Design review of the part built by this model. Coordinates are the model's own, in mm. A direction names the side the tool comes from. Coordinates: 2 decimals unless noted, no trailing zeros. Write each loop counter-clockwise with the first axis right and the second up, starting at its lowest first coordinate (ties: lowest second). Pieces come first, ordered by that corner, then holes.
Q1. Insertion check: pin 1 (2.5 mm diameter, centred on y = 2.5, z = 33.5, fed in from +X); pin 2 (2.5 mm diameter, centred on y = 3, z = -30.5, fed in from +X); pin 3 (0.9 mm diameter, centred on x = -44, z = 25.5, fed in from -Y). Each pin has a flat end and moves straight along its axis. Give the tip position at first contact, or say it passes through.
Q2. Take a section at D-D (y = 1.5). State how many separate pieces and enclosed holes the cut face has, and give its area (3 significant figures).
Q3. Machinability: for faces 1 (the cylindrical face through (-0.325, 1.232, 52.464)), 2 (the cylindrical face through (5.94, 2.46, 42.93)), which of the approach directions +Z, -Z, +X, -X, +Y, -Y give a long, thin tool a straight path to every point of the face, cutting with its end or side? Answer none if there is none.
Q4. Take a section at C-C (z = 19). Give the boundary of the cut face in (x, y).
Q5. Take a section at B-B (x = -30). Give the boundary of the cut face in (y, z).
Q6. For probe 1 along Z at (x, y) = (0, 1.2); probe 2 along X at (y, z) = (4.75, -24); probe 3 along Z at (x, y) = (20, 4.75), list the stretches that pass through material, from the lowest coordinate up.
Q7. Take a section at A-A (x = 0). Give the boundary of the cut face in (y, z), and give its area (3 significant figures).
Q8. Mouldability with a two-part tool opening along X and no side actions: class faces 3 (the cylindrical face through (4.956, 2.465, 23.257)), 4 (the flat face through (-1, 0, -13)) as pulls with the +X half, pulls with the -X half, needs draft (parallel to the pull), parting line crosses it, or undercut.
```python
from build123d import *

# Parameters (mm, degrees)
SKETCH1_R           = 55
BOSS_EXTRUDE1_DEPTH = 5
SKETCH2_R           = 1.5
CUT_EXTRUDE1_DEPTH  = 2.5
SKETCH5_R           = 12.7
CUT_EXTRUDE4_DEPTH  = 6
CUT_EXTRUDE5_DEPTH  = 6
FILLET1_R           = 5
FILLET2_R           = 5


with BuildPart() as part:
    # Sketch1 → Boss-Extrude1 (new body)
    with BuildSketch(Plane(origin=(0, 0, 0), x_dir=(1, 0, 0), z_dir=(0, 1, 0))):
        Circle(SKETCH1_R)
    extrude(amount=BOSS_EXTRUDE1_DEPTH)

    # Sketch2 → Cut-Extrude1 (cut)
    with BuildSketch(Plane(origin=(0, 0, 0), x_dir=(1, 0, 0), z_dir=(0, 1, 0))):
        with Locations((0, 51)):
            Circle(SKETCH2_R)
        with Locations((44.167295593, 25.5)):
            Circle(SKETCH2_R)
        with Locations((44.167295593, -25.5)):
            Circle(SKETCH2_R)
        with Locations((0, -51)):
            Circle(SKETCH2_R)
        with Locations((-44.167295593, -25.5)):
            Circle(SKETCH2_R)
        with Locations((-44.167295593, 25.5)):
            Circle(SKETCH2_R)
    extrude(amount=CUT_EXTRUDE1_DEPTH, mode=Mode.SUBTRACT)

    # Sketch5 → Cut-Extrude4 (cut, through all)
    with BuildSketch(Plane(origin=(0, 5, 0), x_dir=(1, 0, 0), z_dir=(0, 1, 0))):
        Circle(SKETCH5_R)
    extrude(amount=-CUT_EXTRUDE4_DEPTH, mode=Mode.SUBTRACT)

    # Sketch7 → Cut-Extrude5 (cut, through all)
    with BuildSketch(Plane(origin=(0, 5, 0), x_dir=(1, 0, 0), z_dir=(0, 1, 0))):
        with BuildLine():
            Line((-21.351162756, 7.708297411), (-40.816877772, 18.946833216))
            ThreePointArc((-40.816877772, 18.946833216), (-45, 0), (-40.816877772, -18.946833216))
            Line((-40.816877772, -18.946833216), (-21.351162756, -7.708297411))
            ThreePointArc((-21.351162756, -7.708297411), (-22.7, 0), (-21.351162756, 7.708297411))
        make_face()
        with BuildLine():
            Line((-17.351162756, -14.636500641), (-36.816877772, -25.875036446))
            ThreePointArc((-36.816877772, -25.875036446), (-22.5, -38.97114317), (-4, -44.821869662))
            Line((-4, -44.821869662), (-4, -22.344798052))
            ThreePointArc((-4, -22.344798052), (-11.35, -19.658776666), (-17.351162756, -14.636500641))
        make_face()
        with BuildLine():
            ThreePointArc((4, -44.821869662), (22.5, -38.97114317), (36.816877772, -25.875036446))
            Line((36.816877772, -25.875036446), (17.351162756, -14.636500641))
            ThreePointArc((17.351162756, -14.636500641), (11.35, -19.658776666), (4, -22.344798052))
            Line((4, -22.344798052), (4, -44.821869662))
        make_face()
        with BuildLine():
            ThreePointArc((45, 0), (43.941776818, 9.701559159), (40.816877772, 18.946833216))
            Line((40.816877772, 18.946833216), (21.351162756, 7.708297411))
            ThreePointArc((21.351162756, 7.708297411), (22.360248149, 3.912710406), (22.7, 0))
            ThreePointArc((22.7, 0), (22.360248149, -3.912710406), (21.351162756, -7.708297411))
            Line((21.351162756, -7.708297411), (40.816877772, -18.946833216))
            ThreePointArc((40.816877772, -18.946833216), (43.941776818, -9.701559159), (45, 0))
        make_face()
        with BuildLine():
            ThreePointArc((36.816877772, 25.875036446), (22.5, 38.97114317), (4, 44.821869662))
            Line((4, 44.821869662), (4, 22.344798052))
            ThreePointArc((4, 22.344798052), (11.35, 19.658776666), (17.351162756, 14.636500641))
            Line((17.351162756, 14.636500641), (36.816877772, 25.875036446))
        make_face()
        with BuildLine():
            Line((-4, 22.344798052), (-4, 44.821869662))
            ThreePointArc((-4, 44.821869662), (-22.5, 38.97114317), (-36.816877772, 25.875036446))
            Line((-36.816877772, 25.875036446), (-17.351162756, 14.636500641))
            ThreePointArc((-17.351162756, 14.636500641), (-11.35, 19.658776666), (-4, 22.344798052))
        make_face()
    extrude(amount=-CUT_EXTRUDE5_DEPTH, mode=Mode.SUBTRACT)

    # Fillet1
    fillet1_edges = [part.edges().sort_by_distance(p)[0] for p in [
        (-40.816877772, 2.5, -18.946833216),
        (-21.351162756, 2.5, -7.708297411),
        (-21.351162756, 2.5, 7.708297411),
        (-40.816877772, 2.5, 18.946833216),
    ]]
    fillet(fillet1_edges, radius=FILLET1_R)

    # Fillet2
    fillet2_edges = [part.edges().sort_by_distance(p)[0] for p in [
        (40.816877772, 2.5, 18.946833216),
        (21.351162756, 2.5, 7.708297411),
        (21.351162756, 2.5, -7.708297411),
        (40.816877772, 2.5, -18.946833216),
        (36.816877772, 2.5, -25.875036446),
        (17.351162756, 2.5, -14.636500641),
        (4, 2.5, -22.344798052),
        (4, 2.5, -44.821869662),
        (4, 2.5, 44.821869662),
        (4, 2.5, 22.344798052),
        (17.351162756, 2.5, 14.636500641),
        (36.816877772, 2.5, 25.875036446),
        (-36.816877772, 2.5, 25.875036446),
        (-17.351162756, 2.5, 14.636500641),
        (-4, 2.5, 22.344798052),
        (-4, 2.5, 44.821869662),
        (-4, 2.5, -44.821869662),
        (-4, 2.5, -22.344798052),
        (-17.351162756, 2.5, -14.636500641),
        (-36.816877772, 2.5, -25.875036446),
    ]]
    fillet(fillet2_edges, radius=FILLET2_R)


solid = part.part
```
Response:
1. pin 1: stops at x = 44.55
1. pin 2: stops at x = 46.58
1. pin 3: stops at y = 2.5
2. separate pieces: 1
2. enclosed holes: 13
2. area: 5,410 mm2
3. face 1: -Y
3. face 2: +Y, -Y
4. outline: (-51.61, 0) - (-24.91, 0) - (-24.91, 5) - (-51.61, 5) - close; (-12.42, 0) - (12.42, 0) - (12.42, 5) - (-12.42, 5) - close; (24.91, 0) - (51.61, 0) - (51.61, 5) - (24.91, 5) - close
5. outline: (0, -46.1) - (5, -46.1) - (5, -33.54) - (0, -33.54) - close; (0, -21.94) - (5, -21.94) - (5, -12.7) - (0, -12.7) - close; (0, 12.7) - (5, 12.7) - (5, 21.94) - (0, 21.94) - close; (0, 33.54) - (5, 33.54) - (5, 46.1) - (0, 46.1) - close
6. probe 1: z = -55 to -52.5, -49.5 to -12.7, 12.7 to 49.5, 52.5 to 55
6. probe 2: x = -49.49 to -33.03, -4.51 to 4.51, 33.03 to 49.49
6. probe 3: z = -51.23 to -40.31, -16.23 to 16.23, 40.31 to 51.23
7. outline: (0, -55) - (5, -55) - (5, -12.7) - (0, -12.7) - (0, -49.5) - (2.5, -49.5) - (2.5, -52.5) - (0, -52.5) - close; (0, 12.7) - (5, 12.7) - (5, 55) - (0, 55) - (0, 52.5) - (2.5, 52.5) - (2.5, 49.5) - (0, 49.5) - close
7. area: 408 mm2
8. face 3: undercut
8. face 4: needs draft
